from build123d import *

# Parameters (mm, degrees)
F0_R      = 52.5
F0_R_2    = 51
F0_R_3    = 40
F1_DEPTH  = 1
F2_DEPTH  = 5
F3_DEPTH  = 7
F4_W      = 20
F4_H      = 9
F5_DEPTH  = 4.5
F6_R      = 3
F7_DEPTH  = 7.001
F8_W      = 8.0645383788
F8_H      = 6
F9_DEPTH  = 10
F10_R     = 10
F11_DEPTH = 25


with BuildPart() as f1:
    # F0 (on Top) → F1 (new body)
    with BuildSketch(Plane.XY):
        Circle(F0_R)
        Circle(F0_R_2, mode=Mode.SUBTRACT)
        Circle(F0_R_2)
        Circle(F0_R_3, mode=Mode.SUBTRACT)
        Circle(F0_R_3)
    extrude(amount=-F1_DEPTH)

    # F0 (on Top) → F2 (join)
    with BuildSketch(Plane.XY):
        Circle(F0_R_2)
        Circle(F0_R_3, mode=Mode.SUBTRACT)
    extrude(amount=F2_DEPTH)

    # F0 (on Top) → F3 (join)
    with BuildSketch(Plane.XY):
        Circle(F0_R)
        Circle(F0_R_2, mode=Mode.SUBTRACT)
    extrude(amount=F3_DEPTH)

    # F4 (on Top) → F5 (cut)
    with BuildSketch(Plane.XY):
        with Locations((45, 0)):
            Rectangle(F4_W, F4_H)
    extrude(amount=F5_DEPTH, mode=Mode.SUBTRACT)

    # F6 (on Top) → F7 (cut, through all)
    with BuildSketch(Plane.XY):
        with Locations((47.5, 0)):
            Circle(F6_R)
    extrude(amount=F7_DEPTH, mode=Mode.SUBTRACT)

    # F8 (on Top) → F9 (cut)
    with BuildSketch(Plane.XY):
        with Locations((51.5776195013, 0)):
            Rectangle(F8_W, F8_H)
    extrude(amount=F9_DEPTH, mode=Mode.SUBTRACT)

    # F10 (on face) → F11 (join)
    with BuildSketch(Plane.XY):
        Circle(F10_R)
    extrude(amount=F11_DEPTH)


solid = f1.part
The listing builds one solid part. Answer for the finished solid, in the listing's coordinates (mm). A direction names the side the tool comes from. Round coordinates to 2 decimals unless told otherwise and drop trailing zeros. Loops run counter-clockwise (first coordinate to the right, second up) from the corner with the lowest first, then second, coordinate; pieces in that order, holes last. Notation, with made-up numbers: M 49.5,40.5 L 87.5,40.5 A17 ccw 87.5,60.5 Z; hole C 65,-16.75 d9. An arc over 180 degrees is marked long. Write each question's results on one line, items separated by ' | '. Start each with the question number.
1) Determine the mould class of faces 5 (the flat face through (15, -38, 5)), 6 (the flat face through (43, 0, 4.5)), 7 (the cylindrical face through (-2.17, -9.76, 12.32)) for opening direction Z: pulls with the +Z half, pulls with the -Z half, needs draft (parallel to the pull), parting line crosses it, or undercut.
2) Find section D-D on y = -19.5. Write down the section's boundary in (x, z).
3) Find section A-A on y = 0. Write down the section's boundary in (x, z).
4) Straight lines are drawn through the part: probe 1 along Y at (x, z) = (0, 1.25); probe 2 along Y at (x, z) = (0, 6.05); probe 3 along X at (y, z) = (9, 5.75). For each, find the intervals that lie inside material, in ascending order.
5) Find section B-B on z = 2.75. Write down the section's boundary in (x, y).
6) Each of these flat-tipped pins is pushed along its axis until it touches: pin 1 (6 mm diameter, centred on x = -21, z = 12, fed in from -Y); pin 2 (3.5 mm diameter, centred on x = 44, z = 2.5, fed in from +Y); pin 3 (3.5 mm diameter, centred on x = 45, z = 3, fed in from -Y); pin 4 (5 mm diameter, centred on y = 11, z = 4.5, fed in from -X). Where does it stop, or does it pass through?
7) Find section C-C on x = 0. Write down the section's boundary in (y, z), plus the area to 3 significant figures.
8) Which of the six approach directions +Z, -Z, +X, -X, +Y, -Y give full straight-line access (tool end or side, diameter ignored) to faces 1 (the flat face through (46, 4.5, 2)), 2 (the flat face through (51.03, 3, 4.9)), 3 (the cylindrical face through (-8.67, -39.05, 2.46)), 4 (the cylindrical face through (50.076, 15.77, 3.056))?
Final values:
1) face 5: pulls with the +Z half | face 6: undercut | face 7: needs draft
2) outline: M -48.74,-1 L 48.74,-1 L 48.74,7 L 47.12,7 L 47.12,5 L 34.92,5 L 34.92,0 L -34.92,0 L -34.92,5 L -47.12,5 L -47.12,7 L -48.74,7 Z
3) outline: M -52.5,-1 L 52.5,-1 L 52.5,0 L 10,0 L 10,25 L -10,25 L -10,0 L -40,0 L -40,5 L -51,5 L -51,7 L -52.5,7 Z; M 40,4.5 L 44.5,4.5 L 44.5,5 L 40,5 Z
4) probe 1: -52.5 to -40, -10 to 10, 40 to 52.5 | probe 2: -52.5 to -51, -10 to 10, 51 to 52.5 | probe 3: -51.72 to -50.2, -4.36 to 4.36, 50.2 to 51.72
5) outline: C 0,0 d20; M 39.75,-4.5 A40 cw long 39.75,4.5 L 52.31,4.5 A52.5 ccw long 52.31,-4.5 Z
6) pin 1: through | pin 2: y = 31.16 | pin 3: y = -29.76 | pin 4: x = -51.81
7) outline: M -52.5,-1 L 52.5,-1 L 52.5,7 L 51,7 L 51,5 L 40,5 L 40,0 L 10,0 L 10,25 L -10,25 L -10,0 L -40,0 L -40,5 L -51,5 L -51,7 L -52.5,7 Z | area: 736 mm²
8) face 1: +X | face 2: +Z, +X | face 3: +Z | face 4: +Z, -Z
